from build123d import *

# Parameters (mm, degrees)
F0_R      = 1.5
F1_DEPTH  = 1.5
F2_W      = 32.6
F2_H      = 2.5
F3_DEPTH  = 8.5
F4_W      = 6
F4_H      = 8
F5_DEPTH  = 3
F6_W      = 8
F6_H      = 3
F7_DEPTH  = 0.3
F8_R      = 0.4
F9_DEPTH  = 1.5
F10_W     = 8
F10_H     = 2.5
F11_DEPTH = 8.5
F12_W     = 3.25
F12_H     = 16.2
F12_W_2   = 12.5
F13_DEPTH = 13.4
F14_W     = 3.5
F14_H     = 6
F14_W_2   = 10.5
F15_DEPTH = 13.5
F16_W     = 14.6
F16_H     = 14.75
F17_DEPTH = 2
F18_W     = 14.75
F18_H     = 2
F19_DEPTH = 0.1


with BuildPart() as f1:
    # F0 (on Top) → F1 (new body)
    with BuildSketch(Plane.XY):
        with BuildLine():
            Line((-23.1, -23.1), (23.1, -23.1))
            ThreePointArc((23.1, -23.1), (23.807107, -22.807107), (24.1, -22.1))
            Line((24.1, -22.1), (24.1, 22.1))
            ThreePointArc((24.1, 22.1), (23.807107, 22.807107), (23.1, 23.1))
            Line((23.1, 23.1), (-23.1, 23.1))
            ThreePointArc((-23.1, 23.1), (-23.807107, 22.807107), (-24.1, 22.1))
            Line((-24.1, 22.1), (-24.1, -22.1))
            ThreePointArc((-24.1, -22.1), (-23.807107, -22.807107), (-23.1, -23.1))
        make_face()
        with Locations((-21.1, -20.1)):
            Circle(F0_R, mode=Mode.SUBTRACT)
        with Locations((21.1, -20.1)):
            Circle(F0_R, mode=Mode.SUBTRACT)
        with Locations((-21.1, 20.1)):
            Circle(F0_R, mode=Mode.SUBTRACT)
        with Locations((21.1, 20.1)):
            Circle(F0_R, mode=Mode.SUBTRACT)
    extrude(amount=F1_DEPTH)

    # F2 (on face) → F3 (join)
    with BuildSketch(Plane.XY.offset(1.5)):
        with Locations((-0.2, -21.85)):
            Rectangle(F2_W, F2_H)
    extrude(amount=F3_DEPTH)

    # F4 (on face) → F5 (join)
    with BuildSketch(Plane.XY.offset(1.5)):
        with Locations((21.1, -12.6)):
            Rectangle(F4_W, F4_H)
    extrude(amount=F5_DEPTH)

    # F6 (on face) → F7 (join)
    with BuildSketch(Plane.YZ.offset(24.1)):
        with Locations((-12.6, 3)):
            Rectangle(F6_W, F6_H)
    extrude(amount=F7_DEPTH)

    # F8 (on face) → F9 (cut, through all)
    with BuildSketch(Plane.XY.offset(1.5)):
        with Locations((-13, 21.7)):
            Circle(F8_R)
        with Locations((-15.5, 21.7)):
            Circle(F8_R)
        with Locations((-10.5, 21.7)):
            Circle(F8_R)
        with Locations((-8, 21.7)):
            Circle(F8_R)
        with Locations((-5.5, 21.7)):
            Circle(F8_R)
        with Locations((-3, 21.7)):
            Circle(F8_R)
        with Locations((-0.5, 21.7)):
            Circle(F8_R)
        with Locations((2, 21.7)):
            Circle(F8_R)
        with Locations((4.5, 21.7)):
            Circle(F8_R)
        with Locations((7, 21.7)):
            Circle(F8_R)
        with Locations((9.5, 21.7)):
            Circle(F8_R)
        with Locations((12, 21.7)):
            Circle(F8_R)
        with Locations((14.5, 21.7)):
            Circle(F8_R)
        with Locations((14.5, 19.4)):
            Circle(F8_R)
        with Locations((12, 19.4)):
            Circle(F8_R)
        with Locations((9.5, 19.4)):
            Circle(F8_R)
        with Locations((7, 19.4)):
            Circle(F8_R)
        with Locations((4.5, 19.4)):
            Circle(F8_R)
        with Locations((2, 19.4)):
            Circle(F8_R)
        with Locations((-0.5, 19.4)):
            Circle(F8_R)
        with Locations((-3, 19.4)):
            Circle(F8_R)
        with Locations((-5.5, 19.4)):
            Circle(F8_R)
        with Locations((-8, 19.4)):
            Circle(F8_R)
        with Locations((-10.5, 19.4)):
            Circle(F8_R)
        with Locations((-13, 19.4)):
            Circle(F8_R)
        with Locations((-15.5, 19.4)):
            Circle(F8_R)
    extrude(amount=-F9_DEPTH, mode=Mode.SUBTRACT)

    # F10 (on face) → F11 (join)
    with BuildSketch(Plane.XY.offset(1.5)):
        with Locations((-20.1, 13.35)):
            Rectangle(F10_W, F10_H)
    extrude(amount=F11_DEPTH)

    # F12 (on face) → F13 (join)
    with BuildSketch(Plane.XY.offset(1.5)):
        with Locations((-25.725, 0)):
            Rectangle(F12_W, F12_H)
        with Locations((-17.85, 0)):
            Rectangle(F12_W_2, F12_H)
    extrude(amount=F13_DEPTH)

    # F14 (on face) → F15 (join)
    with BuildSketch(Plane.XY.offset(1.5)):
        with Locations((-25.85, -14.1)):
            Rectangle(F14_W, F14_H)
        with Locations((-18.85, -14.1)):
            Rectangle(F14_W_2, F14_H)
    extrude(amount=F15_DEPTH)

    # F16 (on face) → F17 (join)
    with BuildSketch(Plane(origin=(0, 0, 0), x_dir=(1, 0, 0), z_dir=(0, 0, -1))):
        with Locations((16.8, -3.725)):
            Rectangle(F16_W, F16_H)
    extrude(amount=F17_DEPTH)

    # F18 (on face) → F19 (cut)
    with BuildSketch(Plane.YZ.offset(24.1)):
        with Locations((3.725, -1)):
            Rectangle(F18_W, F18_H)
    extrude(amount=-F19_DEPTH, mode=Mode.SUBTRACT)


solid = f1.part
CAD build for the part. Positions are in the model's coordinates, mm. A direction names the side the tool comes from. Round coordinates to 2 decimals unless told otherwise and drop trailing zeros. Write each loop counter-clockwise with the first axis right and the second up, starting at its lowest first coordinate (ties: lowest second). Pieces come first, ordered by that corner, then holes. Notation, with made-up numbers: M 48.5,-7 L 76.5,-7 A19 ccw 76.5,16 Z; hole C 31.25,52.25 d9. An arc over 180 degrees is marked long. Put each result on its own line as item: value. Start each with the question number.
1) Saw through at D-D, the plane x = 19. Write the cut outline in (y, z), and give its area (3 significant figures).
2) Drill centre lines: probe 1 along Y at (x, z) = (-15.5, 0.6); probe 2 along Y at (x, z) = (-17, 3.5); probe 3 along Y at (x, z) = (-12.5, 7.75). Where is each one in solid material? Low to high. Write a range as [from, to].
3) Saw through at A-A, the plane z = 5.25. Write the cut outline in (x, y), and give its area (3 significant figures).
4) 3-axis set-ups, long thin cutter, end or side, ignore diameter. For faces 5 (the flat face through (24, 4, -1)), 6 (the flat face through (-20, 12.1, 6)), 7 (the flat face through (-16.5, -22, 6)), 8 (the flat face through (-21, -11.1, 8)): which of +Z, -Z, +X, -X, +Y, -Y reach the whole face in a straight line?
5) Pull direction X, two halves, no side cores. Call faces 1 (the cylindrical face through (19.6, -20.03, 0.74)), 2 (the flat face through (18.1, -13, 3)), 3 (the flat face through (17, -3.65, -1)), 4 (the flat face through (-16.1, 13, 6)): pulls with the +X half, pulls with the -X half, needs draft (parallel to the pull), parting line crosses it, or undercut.
6) Pin check, flat tips, straight feed: pin 1 Ø4 at (y, z) = (2.5, 6) entering from -X; pin 2 Ø2 at (x, y) = (5, 3.5) entering from -Z; pin 3 Ø3.5 at (x, z) = (22.5, 3.5) entering from +Y; pin 4 Ø2 at (x, z) = (16, -0.5) entering from -Y. Stop position of each tip, or through.
7) Saw through at C-C, the plane y = 4.5. Write the cut outline in (x, z), and give its area (3 significant figures).
8) Saw through at B-B, the plane x = -21.1. Write the cut outline in (y, z).
Resolved:
1. outline: M -23.1,0 L -3.65,0 L -3.65,-2 L 11.1,-2 L 11.1,0 L 23.1,0 L 23.1,1.5 L -8.6,1.5 L -8.6,4.5 L -16.6,4.5 L -16.6,1.5 L -23.1,1.5 Z
1. area: 123 mm²
2. probe 1: [-23.1, 19], [19.8, 21.3], [22.1, 23.1]
2. probe 2: [-17.1, -11.1], [-8.1, 8.1], [12.1, 14.6]
2. probe 3: [-23.1, -20.6], [-8.1, 8.1]
3. outline: M -27.6,-17.1 L -13.6,-17.1 L -13.6,-11.1 L -27.6,-11.1 Z; M -27.35,-8.1 L -11.6,-8.1 L -11.6,8.1 L -27.35,8.1 Z; M -24.1,12.1 L -16.1,12.1 L -16.1,14.6 L -24.1,14.6 Z; M -16.5,-23.1 L 16.1,-23.1 L 16.1,-20.6 L -16.5,-20.6 Z
3. area: 441 mm²
4. face 5: -Z, +X, +Y, -Y
4. face 6: +Z, +X, -X
4. face 7: +Z, -X, -Y
4. face 8: +Z, -X
5. face 1: undercut
5. face 2: undercut
5. face 3: needs draft
5. face 4: pulls with the +X half
6. pin 1: x = -27.35
6. pin 2: z = 0
6. pin 3: y = -8.6
6. pin 4: y = -23.1
7. outline: M -27.35,1.5 L -24.1,1.5 L -24.1,0 L 9.5,0 L 9.5,-2 L 24,-2 L 24,0 L 24.1,0 L 24.1,1.5 L -11.6,1.5 L -11.6,14.9 L -27.35,14.9 Z
7. area: 312 mm²
8. outline: M -23.1,0 L -21.6,0 L -21.6,1.5 L -23.1,1.5 Z; M -18.6,0 L 18.6,0 L 18.6,1.5 L 14.6,1.5 L 14.6,10 L 12.1,10 L 12.1,1.5 L 8.1,1.5 L 8.1,14.9 L -8.1,14.9 L -8.1,1.5 L -11.1,1.5 L -11.1,15 L -17.1,15 L -17.1,1.5 L -18.6,1.5 Z; M 21.6,0 L 23.1,0 L 23.1,1.5 L 21.6,1.5 Z
